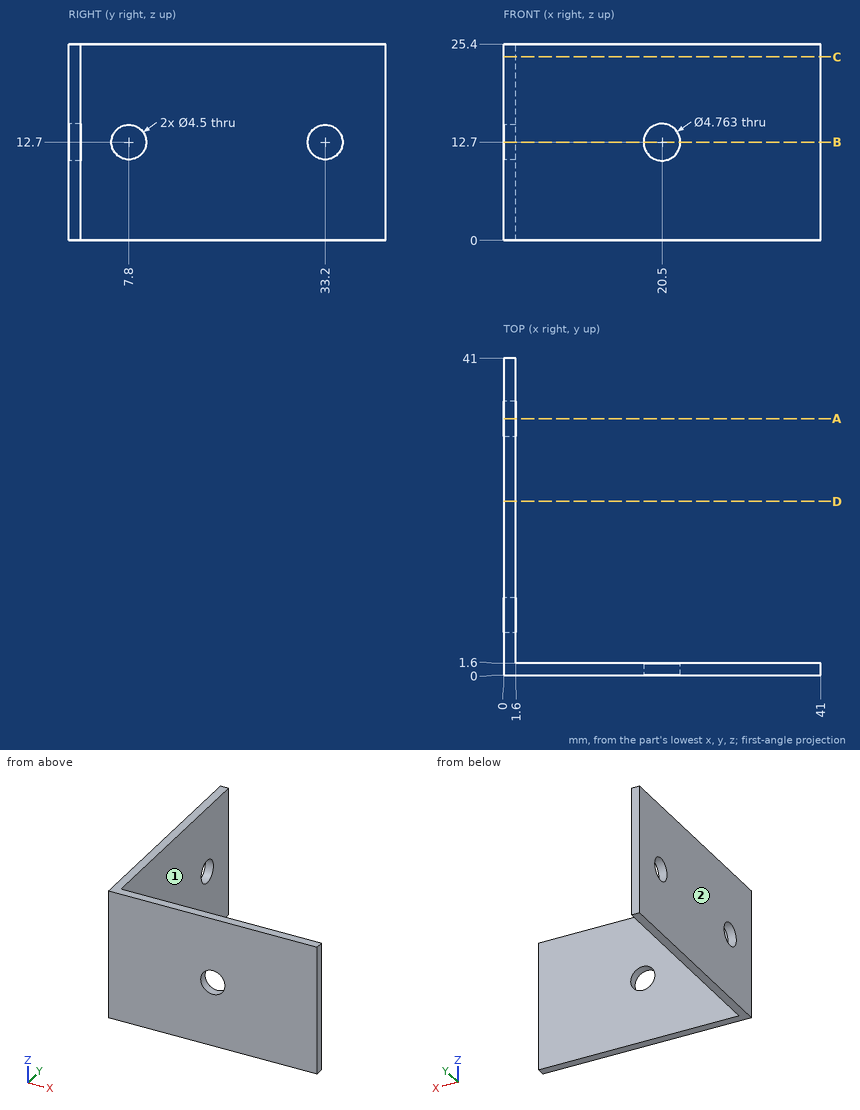
Source: three-view drawing plus pictorial views. Frame: mm from the lowest corner of the part. A direction names the side the tool comes from. Coordinates: 2 decimals unless noted, no trailing zeros. Loops run counter-clockwise (first coordinate to the right, second up) from the corner with the lowest first, then second, coordinate; pieces in that order, holes last. Notation, with made-up numbers: (34, 26.25) - (71, 26.25) arc R25 ccw to (71, 61.25) - close; hole circle Ø7 at (34.5, -18). An arc over 180 degrees is marked (long way). Answer in a Markdown table with one row per item. Add a question column.
Item 1: Section query D-D on y = 22.5. Return the cut outline in (x, z).
Item 2: Line query: line 1 along Z through (x, y) = (20.5, 1.25); line 2 along Z through (x, y) = (0.8, 7.8); line 3 along X through (y, z) = (17, 22.75). Output: solid intervals per line, ascending. Write a range as [from, to].
Item 3: Access query for the marked faces 1 and 2. Directions: +Z, -Z, +X, -X, +Y, -Y. A direction counts if a zero-diameter tool reaches every point of the face in a straight line with its end or side. Return the directions, or none.
Item 4: Section query C-C on z = 23.75. Return the cut outline in (x, y).
Item 5: Section query B-B on z = 12.7. Return the cut outline in (x, y).
Item 6: Contact query for flat-ended pins moving along their axis: P1, Ø2.5, axis at y = 33.2, z = 12.7, coming from the +X side; P2, Ø3, axis at y = 10.5, z = 12, coming from the +X side; P3, Ø8, axis at x = 26.5, z = 9, coming from the +Y side. Output: stop coordinate, or through.
Item 7: Section query A-A on y = 33.2. Return the cut outline in (x, z).
Recorded:
| question | item | result |
|---|---|---|
| 1 | outline | (0, 0) - (1.6, 0) - (1.6, 25.4) - (0, 25.4) - close |
| 2 | line 1 | [0, 10.32], [15.08, 25.4] |
| 2 | line 2 | [0, 10.45], [14.95, 25.4] |
| 2 | line 3 | [0, 1.6] |
| 3 | face 1 | +Z, -Z, +X, +Y |
| 3 | face 2 | +Z, -Z, -X, +Y, -Y |
| 4 | outline | (0, 0) - (41, 0) - (41, 1.6) - (1.6, 1.6) - (1.6, 41) - (0, 41) - close |
| 5 | outline | (0, 0) - (18.12, 0) - (18.12, 1.6) - (1.6, 1.6) - (1.6, 5.55) - (0, 5.55) - close; (0, 10.05) - (1.6, 10.05) - (1.6, 30.95) - (0, 30.95) - close; (0, 35.45) - (1.6, 35.45) - (1.6, 41) - (0, 41) - close; (22.88, 0) - (41, 0) - (41, 1.6) - (22.88, 1.6) - close |
| 6 | P1 | through |
| 6 | P2 | x = 1.6 |
| 6 | P3 | y = 1.6 |
| 7 | outline | (0, 0) - (1.6, 0) - (1.6, 10.45) - (0, 10.45) - close; (0, 14.95) - (1.6, 14.95) - (1.6, 25.4) - (0, 25.4) - close |
